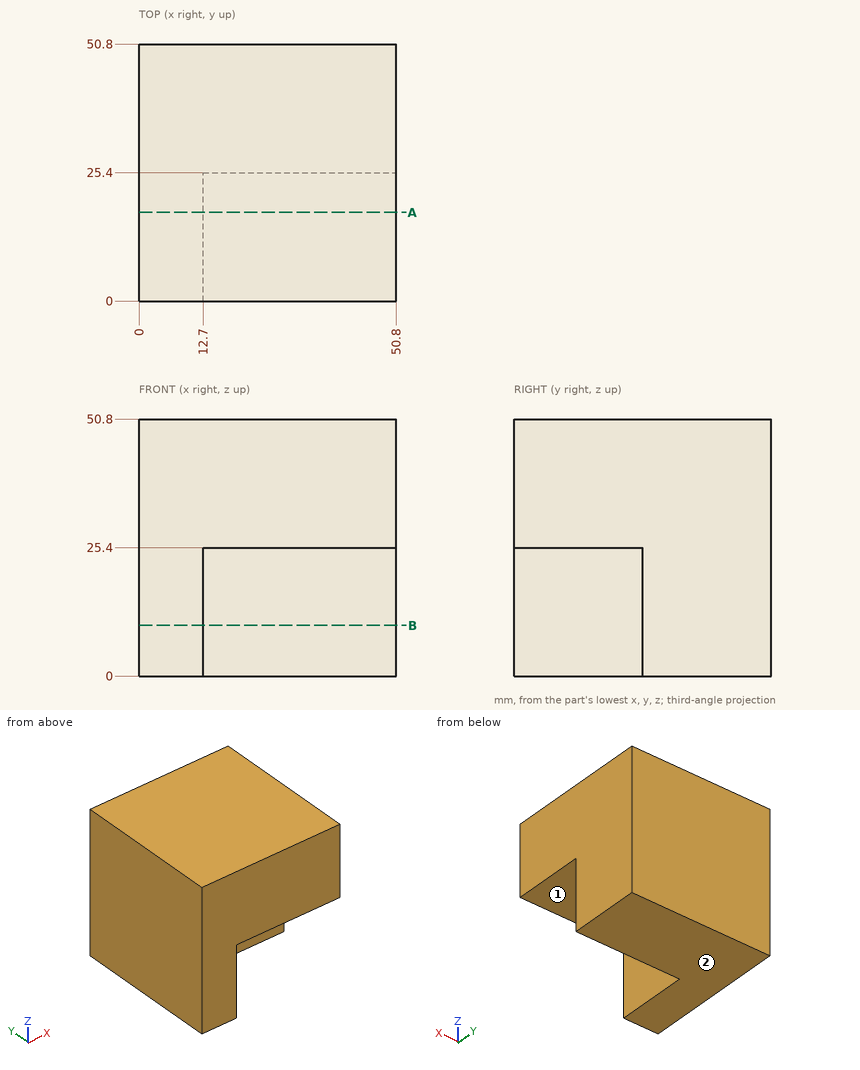
Can you work these out from the drawing? Everything is in mm from the part's minimum corner. A direction names the side the tool comes from. Coordinates: 2 decimals unless noted, no trailing zeros. Order: outer loops, then holes, each group sorted by start corner. A loop starts at its lowest first (then second) coordinate and runs counter-clockwise, first axis right, second up. Notation, with made-up numbers: M -16,63.5 L 13,63.5 A18 cw 13,82.5 Z; hole C -39,30.25 d10. An arc over 180 degrees is marked long. Answer as CSV lines item,"result". Start each with the question number.
1. On a 3-axis mill with a long thin cutter (end or side, diameter ignored), from which of +Z, -Z, +X, -X, +Y, -Y can I reach the whole of each face in a straight line? I mean the marked faces 1 and 2. Say none if no direction works.
2. I want a section at A-A, the plane y = 17.5. Write out the boundary of the cut face in (x, z), and give its area (3 significant figures).
3. I need wall thicknesses on line 1 (Y direction, x = 41.5, z = 17); line 2 (X direction, y = 3.5, z = 4.5). Which ranges of each line are inside material? Lowest first, please. Write a range as [from, to].
4. For pin 1 (3 mm diameter, centred on y = 8.5, z = 10, fed in from +X); pin 2 (7.5 mm diameter, centred on x = 31, z = 10, fed in from -Y), each with a flat end and sliding along its axis, tell me the tip position at first contact or that it passes through.
Recorded:
1,face 1,"-Z, +X, -Y"
1,face 2,"-Z, +X, -X, +Y, -Y"
2,outline,"M 0,0 L 12.7,0 L 12.7,25.4 L 50.8,25.4 L 50.8,50.8 L 0,50.8 Z"
2,area,"1,610 mm2"
3,line 1,"y = [25.4, 50.8]"
3,line 2,"x = [0, 12.7]"
4,pin 1,"stops at x = 12.7"
4,pin 2,"stops at y = 25.4"
